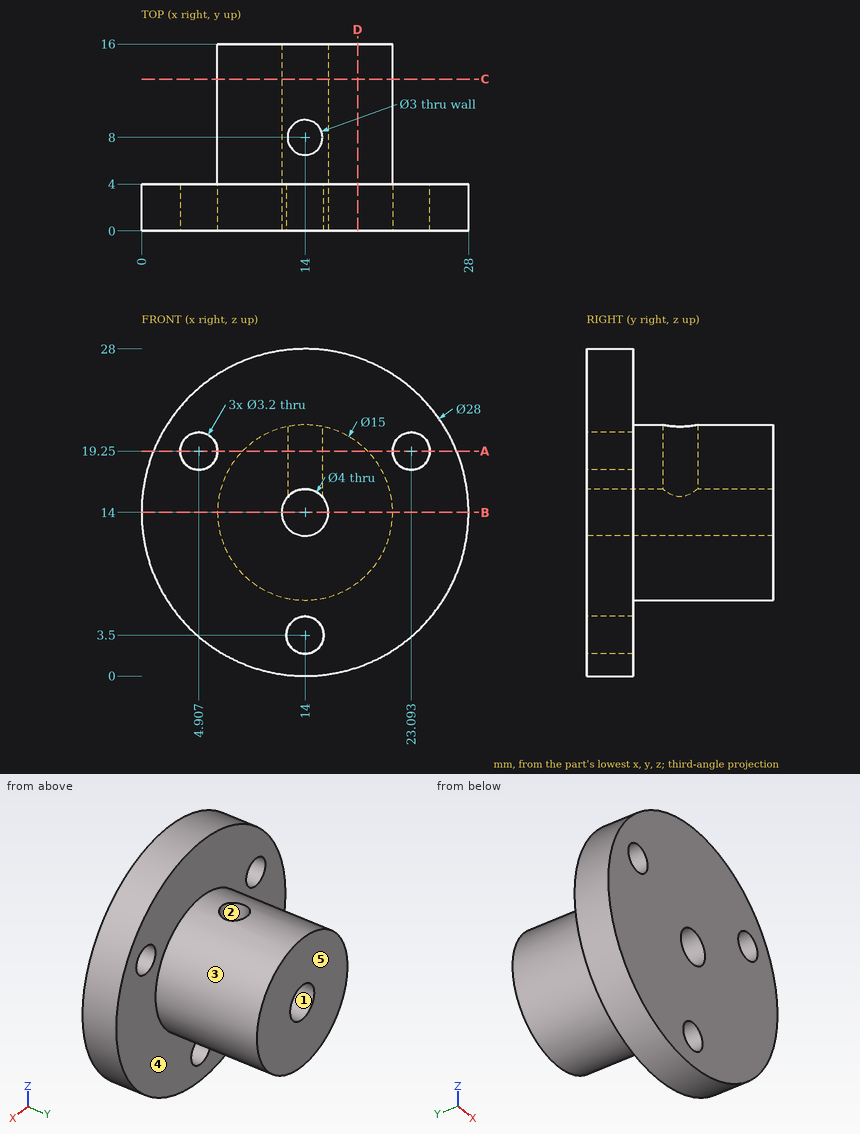
Answer from the drawing. Dimensions are ordinates in mm from the lowest x, y and z of the part. A direction names the side the tool comes from. Round coordinates to 2 decimals unless told otherwise and drop trailing zeros. Loops run counter-clockwise (first coordinate to the right, second up) from the corner with the lowest first, then second, coordinate; pieces in that order, holes last.
1) For a pull along Z with two mould halves and no side action, classify the marked faces 1, 2 and 3 as released by +Z, released by -Z, zero draft, split by the parting line, or undercut.
Outcome:
face 1: undercut
face 2: zero draft
face 3: split by the parting line
2) Consider line 1 (Z direction, x = 14, y = 1.3); line 2 (Y direction, x = 2, z = 7); line 3 (X direction, y = 2.65, z = 19.25). Determine where each line is inside the solid, lowest interval first.
Outcome:
line 1: z = 0 to 1.9, 5.1 to 12, 16 to 28
line 2: y = 0 to 4
line 3: x = 1.02 to 3.31, 6.51 to 21.49, 24.69 to 26.98
3) A cutting plane is placed at C-C on y = 13. Determine the outline of the cut face in (x, z), plus the area to 3 significant figures.
Outcome:
outline: circle Ø15 at (14, 14); hole circle Ø4 at (14, 14)
area: 164 mm2
4) For the marked faces 4 and 5, determine the directions among +Z, -Z, +X, -X, +Y, -Y from which every point of the face is accessible in a straight line to the end or side of a thin tool.
Outcome:
face 4: +Y
face 5: +Z, -Z, +X, -X, +Y
5) A cutting plane is placed at D-D on x = 18.5. Determine the outline of the cut face in (y, z).
Outcome:
outline: (0, 0.74) - (4, 0.74) - (4, 8) - (16, 8) - (16, 20) - (4, 20) - (4, 27.26) - (0, 27.26) - close
6) Given P1, Ø2.5, axis at x = 14, y = 8, coming from the -Z side; P2, Ø4, axis at x = 14, z = 3.5, coming from the -Y side; P3, Ø4, axis at y = 3.5, z = 7, coming from the +X side; P4, Ø3.5, axis at x = 4.91, z = 19.25, coming from the +Y side, each flat-ended and moving along its own axis, determine where each tip first touches the part or whether it passes through.
Outcome:
P1: stops at z = 6.5
P2: stops at y = 0
P3: stops at x = 27.08
P4: stops at y = 4
7) A cutting plane is placed at B-B on z = 14. Determine the outline of the cut face in (x, y).
Outcome:
outline: (0, 0) - (12, 0) - (12, 16) - (6.5, 16) - (6.5, 4) - (0, 4) - close; (16, 0) - (28, 0) - (28, 4) - (21.5, 4) - (21.5, 16) - (16, 16) - close
8) A cutting plane is placed at A-A on z = 19.25. Determine the outline of the cut face in (x, y), plus the area to 3 significant figures.
Outcome:
outline: (1.02, 0) - (3.31, 0) - (3.31, 4) - (1.02, 4) - close; (6.51, 0) - (21.49, 0) - (21.49, 4) - (19.36, 4) - (19.36, 16) - (8.64, 16) - (8.64, 4) - (6.51, 4) - close; (24.69, 0) - (26.98, 0) - (26.98, 4) - (24.69, 4) - close; hole circle Ø3 at (14, 8)
area: 200 mm2
